Design review of the part built by this model. Coordinates are the model's own, in mm. Face numbers are marked on the shaded views. A direction names the side the tool comes from. Coordinates: 2 decimals unless noted, no trailing zeros. Loops run counter-clockwise (first coordinate to the right, second up) from the corner with the lowest first, then second, coordinate; pieces in that order, holes last. Notation, with made-up numbers: (61, -28.5) -> (81, -28.5) arc R22 cw to (81, 8.5) -> close; hole circle Ø10 at (-15.5, 21.25). An arc over 180 degrees is marked (long way). Answer as a JSON object with one key per item and string values.
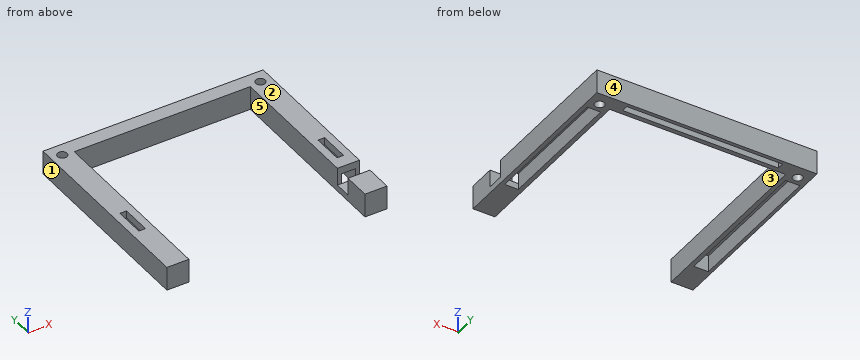
```python
from build123d import *

# Parameters (mm, degrees)
SKETCH2_W           = 150
SKETCH2_H           = 134.5
SKETCH2_W_2         = 120
SKETCH2_H_2         = 114.5
BOSS_EXTRUDE1_DEPTH = 152
SKETCH3_R           = 3.25
CUT_EXTRUDE1_DEPTH  = 27.5
SKETCH4_W           = 120
SKETCH4_H           = 10.090135052
CUT_EXTRUDE2_DEPTH  = 192.859758942
SKETCH5_W           = 9.929816524
SKETCH5_H           = 99.5
SKETCH5_W_2         = 106.146314573
SKETCH5_H_2         = 4.565432885
SKETCH5_W_3         = 9.245001591
CUT_EXTRUDE3_DEPTH  = 140
SKETCH6_W           = 5
SKETCH6_H           = 99.5
BOSS_EXTRUDE2_DEPTH = 10
SKETCH7_W           = 106.146314573
SKETCH7_H           = 5
BOSS_EXTRUDE3_DEPTH = 6
SKETCH8_W           = 5
SKETCH8_H           = 99.5
BOSS_EXTRUDE4_DEPTH = 10
SKETCH9_R           = 3.25
CUT_EXTRUDE4_DEPTH  = 5
SKETCH11_W          = 12
SKETCH11_H          = 11.501568892
CUT_EXTRUDE5_DEPTH  = 35
SKETCH12_W          = 6.942410631
SKETCH12_H          = 9.961568892
BOSS_EXTRUDE5_DEPTH = 9.5
SKETCH13_W          = 4.5
SKETCH13_H          = 20.5
CUT_EXTRUDE6_DEPTH  = 15
SKETCH14_W          = 137.41211241
SKETCH14_H          = 135.633574501
CUT_EXTRUDE7_DEPTH  = 226.792628158


with BuildPart() as part:
    # Sketch2 → Boss-Extrude1 (new body)
    with BuildSketch(Plane.XY):
        with Locations((16.257088332, -6.086968375)):
            Rectangle(SKETCH2_W, SKETCH2_H)
        with Locations((16.257088332, -6.086968375)):
            Rectangle(SKETCH2_W_2, SKETCH2_H_2, mode=Mode.SUBTRACT)
    extrude(amount=BOSS_EXTRUDE1_DEPTH)

    # Sketch3 → Cut-Extrude1 (cut)
    with BuildSketch(Plane.XY.offset(152)):
        with Locations((-51.242911668, 52.163031625)):
            Circle(SKETCH3_R)
        with Locations(Location((83.757088332, 52.163031625, 0), (0, 0, 180))):
            Circle(SKETCH3_R)
    extrude(amount=-CUT_EXTRUDE1_DEPTH, mode=Mode.SUBTRACT)

    # Sketch4 → Cut-Extrude2 (cut, through all)
    with BuildSketch(Plane.XY.offset(152)):
        with Locations((16.257088332, -68.382035901)):
            Rectangle(SKETCH4_W, SKETCH4_H)
    extrude(amount=-CUT_EXTRUDE2_DEPTH, mode=Mode.SUBTRACT)

    # Sketch5 → Cut-Extrude3 (cut)
    with BuildSketch(Plane.XY.offset(152)):
        with Locations((-51.653725831, -3.586968375)):
            Rectangle(SKETCH5_W, SKETCH5_H)
        with Locations((16.314156243, 56.459462148)):
            Rectangle(SKETCH5_W_2, SKETCH5_H_2)
        with Locations((83.825495028, -3.586968375)):
            Rectangle(SKETCH5_W_3, SKETCH5_H)
    extrude(amount=-CUT_EXTRUDE3_DEPTH, mode=Mode.SUBTRACT)

    # Sketch6 → Boss-Extrude2 (add)
    with BuildSketch(Plane.ZY.offset(46.688817569)):
        with Locations((149.5, -3.586968375)):
            Rectangle(SKETCH6_W, SKETCH6_H)
    extrude(amount=BOSS_EXTRUDE2_DEPTH)

    # Sketch7 → Boss-Extrude3 (add)
    with BuildSketch(Plane(origin=(0, 54.176745705, 0), x_dir=(1, 0, 0), z_dir=(0, 1, 0))):
        with Locations((16.314156243, -149.5)):
            Rectangle(SKETCH7_W, SKETCH7_H)
    extrude(amount=BOSS_EXTRUDE3_DEPTH)

    # Sketch8 → Boss-Extrude4 (add)
    with BuildSketch(Plane(origin=(79.202994232, 0, 0), x_dir=(0, 0, -1), z_dir=(1, 0, 0))):
        with Locations((-149.5, -3.586968375)):
            Rectangle(SKETCH8_W, SKETCH8_H)
    extrude(amount=BOSS_EXTRUDE4_DEPTH)

    # Sketch9 → Cut-Extrude4 (cut)
    with BuildSketch(Plane(origin=(0, 0, 0), x_dir=(-1, 0, 0), z_dir=(0, 0, -1))):
        with Locations((-83.757088332, 56.163031625)):
            Circle(SKETCH9_R)
        with Locations((-83.757088332, -3.836968375)):
            Circle(SKETCH9_R)
        with Locations(Location((51.242911668, -3.836968375, 0), (0, 0, 180))):
            Circle(SKETCH9_R)
        with Locations(Location((51.242911668, 56.163031625, 0), (0, 0, 180))):
            Circle(SKETCH9_R)
    extrude(amount=-CUT_EXTRUDE4_DEPTH, mode=Mode.SUBTRACT)

    # Sketch11 → Cut-Extrude5 (cut)
    with BuildSketch(Plane(origin=(91.257088332, 0, 0), x_dir=(0, 0, -1), z_dir=(1, 0, 0))):
        with Locations((-146, -49.126183929)):
            Rectangle(SKETCH11_W, SKETCH11_H)
    extrude(amount=-CUT_EXTRUDE5_DEPTH, mode=Mode.SUBTRACT)

    # Sketch12 → Boss-Extrude5 (add)
    with BuildSketch(Plane(origin=(79.202994232, 0, 0), x_dir=(0, 0, -1), z_dir=(1, 0, 0))):
        with Locations((-136.528794684, -48.356183929)):
            Rectangle(SKETCH12_W, SKETCH12_H)
    extrude(amount=BOSS_EXTRUDE5_DEPTH)

    # Sketch13 → Cut-Extrude6 (cut)
    with BuildSketch(Plane.XY.offset(152)):
        with Locations((83.757088332, -24.266968375)):
            Rectangle(SKETCH13_W, SKETCH13_H)
        with Locations((-51.242911668, -24.266968375)):
            Rectangle(SKETCH13_W, SKETCH13_H)
    extrude(amount=-CUT_EXTRUDE6_DEPTH, mode=Mode.SUBTRACT)

    # Sketch14 → Cut-Extrude7 (cut, through all)
    with BuildSketch(Plane(origin=(91.257088332, 0, 0), x_dir=(0, 0, -1), z_dir=(1, 0, 0))):
        with Locations((-67.050040254, -6.653755626)):
            Rectangle(SKETCH14_W, SKETCH14_H)
    extrude(amount=-CUT_EXTRUDE7_DEPTH, mode=Mode.SUBTRACT)


solid = part.part
```
1) Add section C-C, the plane y = -57. Give the boundary of the cut face in (x, z).
Completed:
{"outline": "(-58.74, 135.76) -> (-43.74, 135.76) -> (-43.74, 152) -> (-58.74, 152) -> close; (76.26, 135.76) -> (91.26, 135.76) -> (91.26, 152) -> (76.26, 152) -> close"}
2) Add section B-B, the plane z = 143.25. Give the boundary of the cut face in (x, y).
Completed:
{"outline": "(-58.74, -73.34) -> (-43.74, -73.34) -> (-43.74, 51.16) -> (76.26, 51.16) -> (76.26, -43.38) -> (79.2, -43.38) -> (79.2, 46.16) -> (88.45, 46.16) -> (88.45, -43.38) -> (91.26, -43.38) -> (91.26, 61.16) -> (-58.74, 61.16) -> close; (76.26, -73.34) -> (91.26, -73.34) -> (91.26, -54.88) -> (76.26, -54.88) -> close; hole (-56.62, -53.34) -> (-46.69, -53.34) -> (-46.69, 46.16) -> (-56.62, 46.16) -> close; hole circle Ø6.5 at (-51.24, 52.16); hole (-36.76, 54.18) -> (69.39, 54.18) -> (69.39, 58.74) -> (-36.76, 58.74) -> close; hole circle Ø6.5 at (83.76, 52.16)"}
3) Add section A-A, the plane y = -28.5. Give the boundary of the cut face in (x, z).
Completed:
{"outline": "(-58.74, 135.76) -> (-56.62, 135.76) -> (-56.62, 147) -> (-53.49, 147) -> (-53.49, 152) -> (-58.74, 152) -> close; (-48.99, 147) -> (-46.69, 147) -> (-46.69, 135.76) -> (-43.74, 135.76) -> (-43.74, 152) -> (-48.99, 152) -> close; (76.26, 135.76) -> (79.2, 135.76) -> (79.2, 147) -> (81.51, 147) -> (81.51, 152) -> (76.26, 152) -> close; (86.01, 147) -> (88.45, 147) -> (88.45, 135.76) -> (91.26, 135.76) -> (91.26, 152) -> (86.01, 152) -> close"}
4) For the marked faces 4 and 5, list the 3-axis set-ups (+Z, -Z, +X, -X, +Y, -Y) from which the entire face can be reached by the end or side of a thin tool; tool diameter is ignored.
Completed:
{"face 4": "+Z, -Z, +X, -X, +Y", "face 5": "+Z, -Z, -Y"}
5) Add section D-D, the plane x = -21. Give the boundary of the cut face in (y, z), and give its area (3 significant figures).
Completed:
{"outline": "(51.16, 135.76) -> (54.18, 135.76) -> (54.18, 147) -> (58.74, 147) -> (58.74, 135.76) -> (61.16, 135.76) -> (61.16, 152) -> (51.16, 152) -> close", "area": "111 mm²"}
6) Clearance check with a flat-ended pin moving along its axis: pin 1 Ø4 at (x, z) = (-18, 146.5) entering from -Y. State where the tip first meets the part, or that it passes through.
Completed:
{"pin 1": "y = 51.16"}
7) The part is to be moulded in two halves that separate along X. For the marked faces 1, 2 and 3, say which applies: pulls with the +X half, pulls with the -X half, needs draft (parallel to the pull), parting line crosses it, or undercut.
Completed:
{"face 1": "pulls with the -X half", "face 2": "needs draft", "face 3": "undercut"}
8) Wall thickness on probe 1 along X at (y, z) = (-38.5, 138.75); probe 2 along X at (y, z) = (-14.5, 149.5); probe 3 along Y at (x, z) = (13, 142.75): over which ranges is each line inside the solid? List them lowest first.
Completed:
{"probe 1": "-58.74 to -56.62, -46.69 to -43.74, 76.26 to 79.2, 88.45 to 91.26", "probe 2": "-58.74 to -53.49, -48.99 to -43.74, 76.26 to 81.51, 86.01 to 91.26", "probe 3": "51.16 to 54.18, 58.74 to 61.16"}
